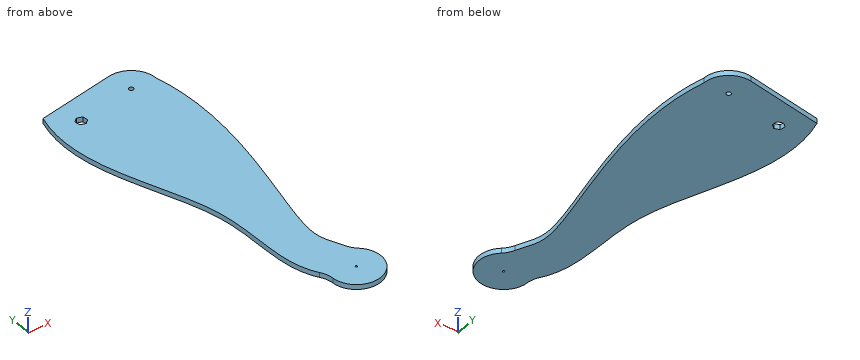
```python
from build123d import *

# Parameters (mm, degrees)
F0_R     = 1
F0_R_2   = 2.35
F2_DEPTH = 5
F3_DEPTH = 5.0010001
F4_R     = 25


with BuildPart() as f2:
    # F0 (on Top) → F2 (new body)
    with BuildSketch(Plane.XY):
        with BuildLine():
            add(Edge.make_bspline(
                [(-82.1230926166, 10.9051483296), (-103.5848878493, -60.0049742057), (-19.3497930189, -169.20375229), (-50.163582636, -268.8476041523), (-24.438918941, -299.5331944222)],
                knots=[0, 0, 0, 0, 0.5562194935, 1, 1, 1, 1], degree=3))
            ThreePointArc((-24.438918941, -299.5331944222), (10.4499069023, -327.5112184995), (11.8990306582, -282.8133433784))
            add(Edge.make_bspline(
                [(25, 0), (47.0782204713, -90.5572716574), (-18.2454262763, -248.1120641616), (7.0555657506, -266.3099283549), (11.8990306582, -282.8133433784)],
                knots=[0, 0, 0, 0, 0.7113740719, 1, 1, 1, 1], degree=3))
            ThreePointArc((25, 0), (16.0696902422, 19.151111078), (-4.3412044417, 24.6201938253))
            Line((-4.3412044417, 24.6201938253), (-82.1230926166, 10.9051483296))
        make_face()
        with Locations((0, -304.8)):
            Circle(F0_R, mode=Mode.SUBTRACT)
        Circle(F0_R_2, mode=Mode.SUBTRACT)
    extrude(amount=F2_DEPTH)

    # F1 (on Top) → F3 (cut, through all)
    with BuildSketch(Plane.XY):
        Polygon((-53.9344131989, -12.2948121673), (-54.886843509, -6.8933114649), (-60.0408954909, -5.0173899577), (-64.2425171626, -8.5429691528), (-63.2900868525, -13.9444698551), (-58.1360348706, -15.8203913624), align=None)
    extrude(amount=F3_DEPTH, mode=Mode.SUBTRACT)

    # F4
    f4_edges = [f2.edges().sort_by_distance(p)[0] for p in [
        (-24.438919, -299.533194, 2.5),
        (11.899031, -282.813343, 2.5),
    ]]
    fillet(f4_edges, radius=F4_R)


solid = f2.part
```
For this review, take the finished solid that the model builds, in its own axes (mm). Round coordinates to 2 decimals unless told otherwise and drop trailing zeros. Use one line per item in the form item = value.
1) Take a section at A-A, the plane z = 2.9. Count the separate pieces of the cut face and the enclosed holes in it, and give its area (3 significant figures).
Found:
separate_pieces = 1
enclosed_holes = 3
area = 26,300 mm2
2) Clearance check with flat-ended pins moving along their axes: pin 1 (3 mm diameter, centred on x = -36, z = 4, fed in from -Y); pin 2 (8 mm diameter, centred on x = -36, y = -253.5, fed in from -Z); pin 3 (3 mm diameter, centred on y = -131.5, z = 3.5, fed in from -X); pin 4 (1.5 mm diameter, centred on y = -60.5, z = 3.5, fed in from -X). State where each tip first meets the part, or that it passes through.
Found:
pin_1 = -282.64
pin_2 = 0
pin_3 = -60.69
pin_4 = -84.09
3) To check wall thickness, follow L1, parallel to X at y = -304.8, z = 1.45; L2, parallel to X at y = -17, z = 1.5; L3, parallel to Y at x = -30.5, z = 0.7. State the ranges of each line that lie inside material, in increasing order. Write a range as from..to.
Found:
L1 = -25.05..-1, 1..25
L2 = -87.32..28.33
L3 = -290.88..20.01
